Work out the finished part from the listing and answer in its coordinate system (mm). Face numbers are marked on the shaded views. A direction names the side the tool comes from. Round coordinates to 2 decimals unless told otherwise and drop trailing zeros. Loops run counter-clockwise (first coordinate to the right, second up) from the corner with the lowest first, then second, coordinate; pieces in that order, holes last.
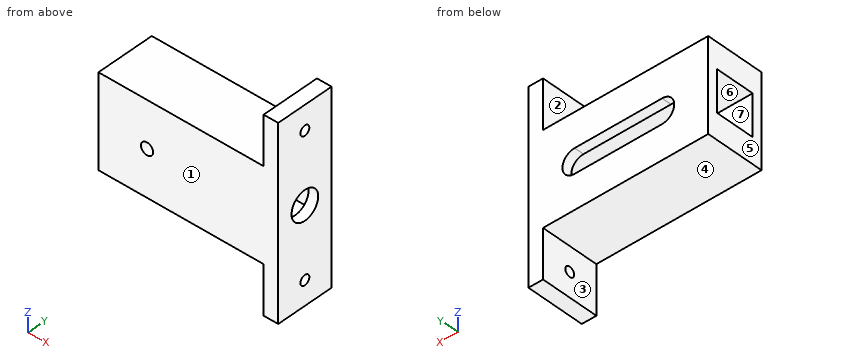
```python
from build123d import *

# Parameters (mm, degrees)
CROQUIS1_W              = 33
CROQUIS1_H              = 15
CROQUIS1_W_2            = 2
SALIENTE_EXTRUIR1_DEPTH = 2
SALIENTE_EXTRUIR2_DEPTH = 10
CROQUIS2_W              = 37
CROQUIS2_H              = 19
SALIENTE_EXTRUIR3_DEPTH = 2
CORTAR_EXTRUIR4_DEPTH   = 3
CROQUIS8_W              = 3
CROQUIS8_H              = 12
SALIENTE_EXTRUIR5_DEPTH = 10
CROQUIS9_R              = 1
CORTAR_EXTRUIR5_DEPTH   = 10
CROQUIS10_W             = 3.25
CROQUIS10_H             = 8
SALIENTE_EXTRUIR6_DEPTH = 35
CROQUIS11_R             = 3
CORTAR_EXTRUIR6_DEPTH   = 35
CROQUIS12_R             = 1.25
CORTAR_EXTRUIR7_DEPTH   = 5


with BuildPart() as part:
    # Croquis1 → Saliente-Extruir1 (new body)
    with BuildSketch(Plane(origin=(0, 0, 0), x_dir=(1, 0, 0), z_dir=(0, 1, 0))):
        Rectangle(CROQUIS1_W, CROQUIS1_H)
        with Locations((-17.5, 0)):
            Rectangle(CROQUIS1_W_2, CROQUIS1_H)
    extrude(amount=SALIENTE_EXTRUIR1_DEPTH)

    # Croquis1_4 → Saliente-Extruir2 (add)
    with BuildSketch(Plane(origin=(0, 0, 0), x_dir=(1, 0, 0), z_dir=(0, 1, 0))):
        Polygon((16.5, -7.5), (-16.5, -7.5), (-18.5, -7.5), (-18.5, -9.5), (18.5, -9.5), (18.5, 9.5), (-18.5, 9.5), (-18.5, 7.5), (-16.5, 7.5), (16.5, 7.5), align=None)
    extrude(amount=SALIENTE_EXTRUIR2_DEPTH)

    # Croquis2 → Saliente-Extruir3 (add)
    with BuildSketch(Plane(origin=(0, 10, 0), x_dir=(1, 0, 0), z_dir=(0, 1, 0))):
        Rectangle(CROQUIS2_W, CROQUIS2_H)
    extrude(amount=SALIENTE_EXTRUIR3_DEPTH)

    # Croquis7 → Cortar-Extruir4 (cut)
    with BuildSketch(Plane(origin=(0, 12, 0), x_dir=(1, 0, 0), z_dir=(0, 1, 0))):
        with BuildLine():
            Line((-9, 2.5), (9, 2.5))
            ThreePointArc((9, 2.5), (11.5, 0), (9, -2.5))
            Line((9, -2.5), (-9, -2.5))
            ThreePointArc((-9, -2.5), (-11.5, 0), (-9, 2.5))
        make_face()
    extrude(amount=-CORTAR_EXTRUIR4_DEPTH, mode=Mode.SUBTRACT)

    # Croquis8 → Saliente-Extruir5 (add)
    with BuildSketch(Plane(origin=(0, 0, -9.5), x_dir=(-1, 0, 0), z_dir=(0, 0, -1))):
        with Locations((-17, 6)):
            Rectangle(CROQUIS8_W, CROQUIS8_H)
    saliente_extruir5 = extrude(amount=SALIENTE_EXTRUIR5_DEPTH)

    # Croquis9 → Cortar-Extruir5 (cut)
    with BuildSketch(Plane.ZY.offset(-15.5)):
        with Locations((-14.5, 6)):
            Circle(CROQUIS9_R)
    cortar_extruir5 = extrude(amount=-CORTAR_EXTRUIR5_DEPTH, mode=Mode.SUBTRACT)

    # Simetr_a3: Saliente-Extruir5, Cortar-Extruir5 across plane
    add(saliente_extruir5.mirror(Plane.XY))
    add(cortar_extruir5.mirror(Plane.XY), mode=Mode.SUBTRACT)

    # Croquis10 → Saliente-Extruir6 (add)
    with BuildSketch(Plane.ZY.offset(-16.5)):
        with Locations((-5.875, 6)):
            Rectangle(CROQUIS10_W, CROQUIS10_H)
        with Locations((5.875, 6)):
            Rectangle(CROQUIS10_W, CROQUIS10_H)
    extrude(amount=SALIENTE_EXTRUIR6_DEPTH)

    # Croquis11 → Cortar-Extruir6 (cut)
    with BuildSketch(Plane(origin=(18.5, 0, 0), x_dir=(0, 0, -1), z_dir=(1, 0, 0))):
        with Locations((0, 6)):
            Circle(CROQUIS11_R)
    extrude(amount=-CORTAR_EXTRUIR6_DEPTH, mode=Mode.SUBTRACT)

    # Croquis12 → Cortar-Extruir7 (cut)
    with BuildSketch(Plane.XZ):
        with Locations(Location((-8.5, 0, 0), (0, 0, 270))):
            Circle(CROQUIS12_R)
    extrude(amount=-CORTAR_EXTRUIR7_DEPTH, mode=Mode.SUBTRACT)


solid = part.part
```
1. Given pin 1 (4 mm diameter, centred on x = -9.5, y = 5.5, fed in from -Z); pin 2 (2 mm diameter, centred on x = 2, y = 11, fed in from +Z), each flat-ended and moving along its own axis, determine where each tip first touches the part or whether it passes through.
Answer key:
pin 1: stops at z = -9.5
pin 2: stops at z = 9.5
2. Determine the mould class of the marked faces 4, 5, 6 and 7 for opening direction Z: +Z half, -Z half, draft (parallel to the pull), parting line (faces both ways), or undercut.
Answer key:
face 4: -Z half
face 5: draft
face 6: undercut
face 7: undercut
3. Which of the six approach directions +Z, -Z, +X, -X, +Y, -Y give full straight-line access (tool end or side, diameter ignored) to the marked faces 1, 2 and 3?
Answer key:
face 1: +Z, -Z, +X, -X, -Y
face 2: +Z, -X, +Y, -Y
face 3: -Z, -X, +Y, -Y
4. Find section A-A (z = 14.5). Write down the section's boundary in (x, y), then the cut area to 3 significant figures.
Answer key:
outline: (15.5, 0) - (18.5, 0) - (18.5, 5) - (15.5, 5) - close; (15.5, 7) - (18.5, 7) - (18.5, 12) - (15.5, 12) - close
area: 30.0 mm2
5. Consider probe 1 along Z at (x, y) = (9, 7.75); probe 2 along X at (y, z) = (1.25, 0); probe 3 along Z at (x, y) = (12, 0.5). Determine where each line is inside the solid, lowest interval first.
Answer key:
probe 1: z = -9.5 to -4.25, 4.25 to 9.5
probe 2: x = -18.5 to -9.75, -7.25 to 18.5
probe 3: z = -9.5 to 9.5
6. Find section C-C (y = 1.5). Write down the section's boundary in (x, z).
Answer key:
outline: (-18.5, -9.5) - (15.5, -9.5) - (15.5, -19.5) - (18.5, -19.5) - (18.5, 19.5) - (15.5, 19.5) - (15.5, 9.5) - (-18.5, 9.5) - close; hole circle Ø2.5 at (-8.5, 0)
7. Find section D-D (y = 6). Write down the section's boundary in (x, z).
Answer key:
outline: (-18.5, -9.5) - (15.5, -9.5) - (15.5, -13.5) - (18.5, -13.5) - (18.5, -3) - (16.5, -3) - (16.5, -4.25) - (-18.5, -4.25) - close; (-18.5, 4.25) - (16.5, 4.25) - (16.5, 3) - (18.5, 3) - (18.5, 13.5) - (15.5, 13.5) - (15.5, 9.5) - (-18.5, 9.5) - close; (15.5, -19.5) - (18.5, -19.5) - (18.5, -15.5) - (15.5, -15.5) - close; (15.5, 15.5) - (18.5, 15.5) - (18.5, 19.5) - (15.5, 19.5) - close
8. Find section B-B (x = -8.5). Write down the section's boundary in (y, z).
Answer key:
outline: (0, -9.5) - (12, -9.5) - (12, -2.5) - (10, -2.5) - (10, -4.25) - (2, -4.25) - (2, -1.25) - (0, -1.25) - close; (0, 1.25) - (2, 1.25) - (2, 4.25) - (10, 4.25) - (10, 2.5) - (12, 2.5) - (12, 9.5) - (0, 9.5) - close
